from build123d import *

# Parameters (mm, degrees)
SKETCH1_W           = 50
SKETCH1_H           = 20
BOSS_EXTRUDE1_DEPTH = 2
SKETCH2_W           = 10
SKETCH2_H           = 2
BOSS_EXTRUDE2_DEPTH = 18
FILLET1_SIZE        = 10
FILLET1_SIZE_2      = 18
FILLET2_SIZE        = 18
FILLET2_SIZE_2      = 10
CUT_EXTRUDE1_DEPTH  = 33.388269589
SKETCH5_R           = 1.75
CUT_EXTRUDE2_DEPTH  = 33.388269589
SKETCH6_R           = 2
CUT_EXTRUDE3_DEPTH  = 37.728735461


with BuildPart() as part:
    # Sketch1 → Boss-Extrude1 (new body)
    with BuildSketch(Plane(origin=(0, 0, 0), x_dir=(1, 0, 0), z_dir=(0, 1, 0))):
        Rectangle(SKETCH1_W, SKETCH1_H)
    extrude(amount=BOSS_EXTRUDE1_DEPTH)

    # Sketch2 → Boss-Extrude2 (add)
    with BuildSketch(Plane(origin=(0, 2, 0), x_dir=(1, 0, 0), z_dir=(0, 1, 0))):
        with Locations((-20, 9)):
            Rectangle(SKETCH2_W, SKETCH2_H)
        with Locations((20, 9)):
            Rectangle(SKETCH2_W, SKETCH2_H)
    extrude(amount=BOSS_EXTRUDE2_DEPTH)

    # Fillet1
    # an asymmetric fillet: 18, 10 mm, written as the material it takes off along each edge
    with BuildSketch(Plane(origin=(-25, -45, 10), x_dir=(1, 0, 0), z_dir=(0, 1, 0))) as fillet1_piece_1:
        with BuildLine():
            Bezier((FILLET1_SIZE, 0), (0, 0), (0, FILLET1_SIZE_2), weights=[1, 0.707106781, 1])
            Line((0, FILLET1_SIZE_2), (0, 0))
            Line((0, 0), (FILLET1_SIZE, 0))
        make_face()
    extrude(amount=92, mode=Mode.SUBTRACT)

    # Fillet2
    # an asymmetric fillet: 18, 10 mm, written as the material it takes off along each edge
    with BuildSketch(Plane(origin=(25, -45, 10), x_dir=(0, 0, -1), z_dir=(0, 1, 0))) as fillet2_piece_1:
        with BuildLine():
            Bezier((FILLET2_SIZE, 0), (0, 0), (0, FILLET2_SIZE_2), weights=[1, 0.707106781, 1])
            Line((0, FILLET2_SIZE_2), (0, 0))
            Line((0, 0), (FILLET2_SIZE, 0))
        make_face()
    extrude(amount=92, mode=Mode.SUBTRACT)

    # Sketch4 → Cut-Extrude1 (cut, through all)
    with BuildSketch(Plane(origin=(0, 2, 0), x_dir=(1, 0, 0), z_dir=(0, 1, 0))):
        with BuildLine():
            Line((-6, 7.5), (-6, 10))
            Line((-6, 10), (6, 10))
            Line((6, 10), (6, 7.5))
            ThreePointArc((6, 7.5), (0, 1.5), (-6, 7.5))
        make_face()
    extrude(amount=-CUT_EXTRUDE1_DEPTH, mode=Mode.SUBTRACT)

    # Sketch5 → Cut-Extrude2 (cut, through all)
    with BuildSketch(Plane(origin=(0, 2, 0), x_dir=(1, 0, 0), z_dir=(0, 1, 0))):
        with Locations(Location((-9, 7.5, 0), (0, 0, 270))):
            Circle(SKETCH5_R)
        with Locations(Location((9, 7.5, 0), (0, 0, 270))):
            Circle(SKETCH5_R)
    extrude(amount=-CUT_EXTRUDE2_DEPTH, mode=Mode.SUBTRACT)

    # Sketch6 → Cut-Extrude3 (cut, through all)
    with BuildSketch(Plane.XY.offset(-8)):
        with Locations((20, 11)):
            Circle(SKETCH6_R)
        with Locations((-20, 11)):
            Circle(SKETCH6_R)
    extrude(amount=-CUT_EXTRUDE3_DEPTH, mode=Mode.SUBTRACT)


solid = part.part
The listing builds one solid part. Answer for the finished solid, in the listing's coordinates (mm). A direction names the side the tool comes from. Give positions to 0.01 mm unless a question says otherwise; leave off trailing zeros. Write each loop counter-clockwise with the first axis right and the second up, starting at its lowest first coordinate (ties: lowest second). Pieces come first, ordered by that corner, then holes.
Item 1: Determine the mould class of faces 4 (the flat face through (-22.3, 10.9, -8)), 5 (the flat face through (-25, 10, -9)), 6 (the cylindrical face through (-20, 13, -9)) for opening direction X: released by +X, released by -X, zero draft, split by the parting line, or undercut.
Item 2: Section B-B, the plane y = 3.5 is taken. Write down the section's boundary in (x, z).
Item 3: Which of the six approach directions +Z, -Z, +X, -X, +Y, -Y give full straight-line access (tool end or side, diameter ignored) to faces 1 (the flat face through (6, 1, -9)), 2 (the flat face through (15, 11, -9)), 3 (the flat face through (17.7, 10.9, -8))?
Item 4: Section C-C, the plane x = 0 is taken. Write down the section's boundary in (y, z), plus the area to 3 significant figures.
Item 5: Flat-ended cylindrical pins translate along their axes: P1, Ø6, axis at x = 7.5, z = -3.5, coming from the +Y side; P2, Ø5, axis at x = -17.5, y = 4, coming from the +Z side; P3, Ø11, axis at x = 19, y = 10, coming from the +Z side. Find the tip coordinate at first contact, or state that the pin passes through.
Item 6: Find the intervals of material crossed by line 1 along X through (y, z) = (0.9, -7.5); line 2 along X through (y, z) = (3.5, -8.75); line 3 along Z through (x, y) = (22, 14.5), in increasing order.
Item 7: Section A-A, the plane x = 9 is taken. Write down the section's boundary in (y, z).
Completed:
1. face 4: zero draft
1. face 5: released by -X
1. face 6: undercut
2. outline: (-25, -10) - (-15, -10) - (-15, -8) - (-25, -8) - close; (15, -10) - (25, -10) - (25, -8) - (15, -8) - close
3. face 1: -Z, +Y, -Y
3. face 2: +Z, -Z, +Y
3. face 3: +Z, +X, -X, +Y
4. outline: (0, -1.5) - (2, -1.5) - (2, 10) - (0, 10) - close
4. area: 23.0 mm2
5. P1: stops at y = 2
5. P2: stops at z = 9.91
5. P3: stops at z = -8
6. line 1: x = -25 to -10.75, -7.25 to -6, 6 to 7.25, 10.75 to 25
6. line 2: x = -25 to -15, 15 to 25
6. line 3: z = -10 to -8
7. outline: (0, -10) - (2, -10) - (2, -9.25) - (0, -9.25) - close; (0, -5.75) - (2, -5.75) - (2, 10) - (0, 10) - close
